Autodesk Inventor part; units mm, degrees
ref_plane "YZ Plane" through (0, 0, 0) normal (1, 0, 0) x (0, 1, 0)
ref_plane "XZ Plane" through (0, 0, 0) normal (0, 1, 0) x (-1, 0, 0)
ref_plane "XY Plane" through (0, 0, 0) normal (0, 0, 1) x (1, 0, 0)
sketch "Sketch1" plane through (0, 0, 0) normal (0, 1, 0) x (-1, 0, 0)
  point P0 (0, 0)
sketch "Sketch2" plane through (0, 0, 0) normal (0, 1, 0) x (-1, 0, 0)
  line L0 (0, 0) -> (76, 0)
  line L1 (76, 0) -> (76, -76)
  line L2 (76, -76) -> (0, -76)
  line L3 (0, -76) -> (0, 0)
  dimension "d3" = 76
  dimension "d4" = 76
extrude "Extrusion1" add sketch "Sketch2" along normal blind 42.6
sketch "Sketch3" plane through (0, 42.6, 0) normal (0, 1, 0) x (1, 0, 0)
  circle A0 centre (-38, 38) radius 25
  point P0 (0, 0)
  dimension "d7" = 50
extrude "Extrusion2" add sketch "Sketch3" along normal blind 5.1
sketch "Sketch4" plane through (-38, 47.7, -38) normal (0, 1, 0) x (1, 0, 0)
  circle A0 centre (0, 0) radius 23
  point P0 (38, -38)
  dimension "d10" = 46
extrude "Extrusion3" add sketch "Sketch4" along normal blind 3.8
sketch "Sketch5" plane through (-38, 51.5, -38) normal (0, 1, 0) x (1, 0, 0)
  circle A0 centre (0, 0) radius 25
  point P0 (38, -38)
extrude "Extrusion4" add sketch "Sketch5" along normal blind 6.1
sketch "Sketch6" plane through (0, 0, 0) normal (0, -1, 0) x (1, 0, 0)
  circle A0 centre (-38, -38) radius 19
  point P0 (0, 0)
  dimension "d15" = 38
extrude "Extrusion5" cut sketch "Sketch6" against normal blind 8.1
sketch "Sketch7" plane through (-38, 8.1, -38) normal (0, -1, 0) x (1, 0, 0)
  circle A0 centre (0, 0) radius 14.2
  point P0 (38, 38)
  dimension "d18" = 28.4
extrude "Extrusion6" cut sketch "Sketch7" against normal blind 7
sketch "Sketch8" plane through (-38, 15.1, -38) normal (0, -1, 0) x (1, 0, 0)
  circle A0 centre (0, 0) radius 16.5
  point P0 (38, 38)
  dimension "d21" = 33
extrude "Extrusion7" cut sketch "Sketch8" against normal blind 12.5
sketch "Sketch9" plane through (-38, 57.6, -38) normal (0, 1, 0) x (1, 0, 0)
  circle A0 centre (0, 0) radius 14.2
  point P0 (38, -38)
  dimension "d24" = 28.4
extrude "Extrusion8" cut sketch "Sketch9" against normal blind 30
The listing builds one solid part. Answer for the finished solid, in the listing's coordinates (mm). A direction names the side the tool comes from. Give positions to 0.01 mm unless a question says otherwise; leave off trailing zeros. Order: outer loops, then holes, each group sorted by start corner. A loop starts at its lowest first (then second) coordinate and runs counter-clockwise, first axis right, second up. Notation, with made-up numbers: (82, 10.25) -> (115, 10.25) arc R28 cw to (115, 38.25) -> close; hole circle Ø10 at (22.5, 23.25). An arc over 180 degrees is marked (long way). Answer as a JSON object with one key per item and string values. Group by question number.
Item 1: Determine the mould class of faces 5 (the flat face through (-27, 57.6, -27)), 6 (the flat face through (-31, 8.1, -51)), 7 (the cylindrical face through (-58, 45, -53)) for opening direction X: pulls with the +X half, pulls with the -X half, needs draft (parallel to the pull), parting line crosses it, or undercut.
Item 2: A flat-ended cylindrical pin translates along its axis: pin 1 (1.5 mm diameter, centred on y = 43.5, z = -37, fed in from -X). Find the tip coordinate at first contact, or state that the pin passes through.
Item 3: The part is cut by section D-D on z = -58. Write down the section's boundary in (x, y), and give its area (3 significant figures).
Item 4: Consider L1, parallel to Z at x = -38, y = 54; L2, parallel to X at y = 36, z = -38; L3, parallel to Z at x = -38, y = 18.25. Determine where each line is inside the solid, lowest interval first. Write a range as from..to.
Item 5: The part is cut by section C-C on y = 29. Write down the section's boundary in (x, z), and give its area (3 significant figures).
Item 6: A tool of negligible diameter and unlimited length cuts with its end or side. For faces 1 (the flat face through (-37, 21, 0)), 2 (the cylindrical face through (-58, 55, -53)), 3 (the cylindrical face through (-42.119, 3.993, -56.548)), 4 (the cylindrical face through (-16.062, 49.573, -31.091)), from which of +Z, -Z, +X, -X, +Y, -Y can it reach the whole face along a straight path? Write none if from no direction.
Result set:
{
 "1": {"face 5": "needs draft", "face 6": "undercut", "face 7": "parting line crosses it"},
 "2": {"pin 1": "x = -63"},
 "3": {"outline": "(-76, 0) -> (0, 0) -> (0, 42.6) -> (-23, 42.6) -> (-23, 47.7) -> (-26.64, 47.7) -> (-26.64, 51.5) -> (-23, 51.5) -> (-23, 57.6) -> (-53, 57.6) -> (-53, 51.5) -> (-49.36, 51.5) -> (-49.36, 47.7) -> (-53, 47.7) -> (-53, 42.6) -> (-76, 42.6) -> close", "area": "3,660 mm²"},
 "4": {"L1": "-63..-52.2, -23.8..-13", "L2": "-76..-52.2, -23.8..0", "L3": "-76..-54.5, -21.5..0"},
 "5": {"outline": "(-76, -76) -> (0, -76) -> (0, 0) -> (-76, 0) -> close; hole circle Ø28.4 at (-38, -38)", "area": "5,140 mm²"},
 "6": {"face 1": "+Z, +X, -X, +Y, -Y", "face 2": "+Y", "face 3": "-Y", "face 4": "none"}
}
